The figure shows three views and two pictorial views of one solid part (mm, origin at its lowest corner). Answer the questions. A direction names the side the tool comes from. Round coordinates to 2 decimals unless told otherwise and drop trailing zeros. Order: outer loops, then holes, each group sorted by start corner. A loop starts at its lowest first (then second) coordinate and runs counter-clockwise, first axis right, second up. Notation, with made-up numbers: (38, 79) - (46, 79) arc R13 cw to (46, 95) - close; hole circle Ø5 at (77.5, 38). An arc over 180 degrees is marked (long way). Write item = value, one per line.
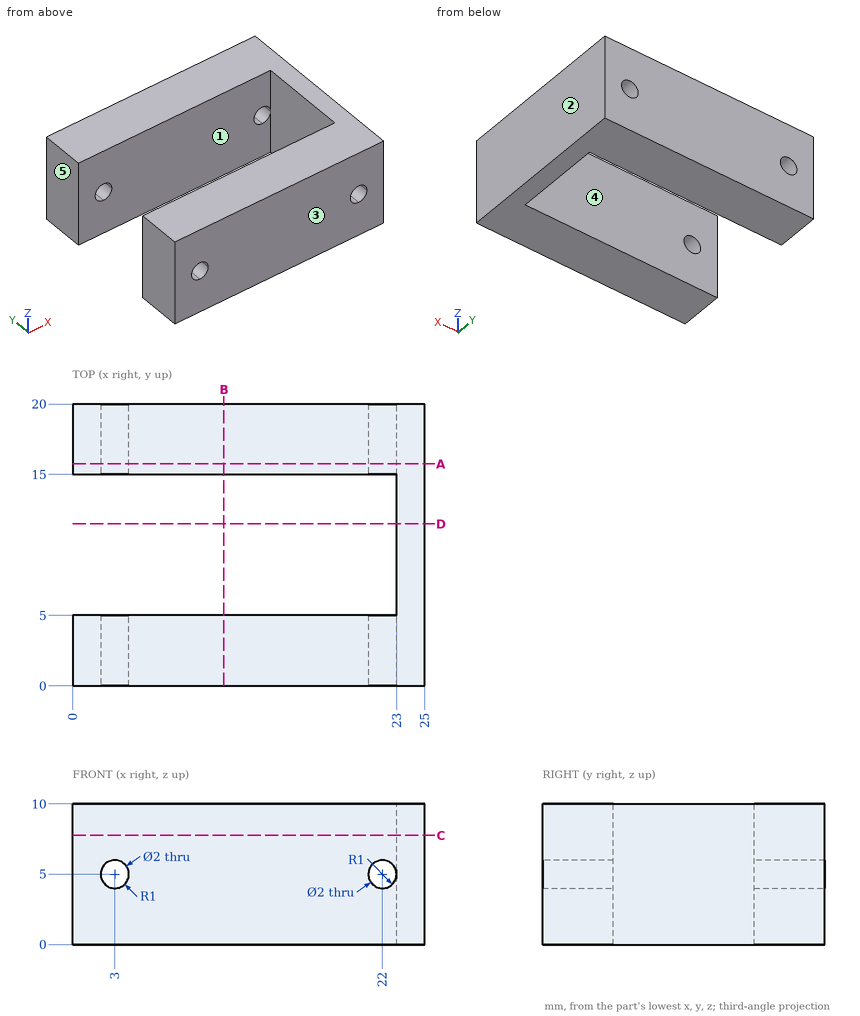
Q1. Determine the mould class of the marked faces 3, 4 and 5 for opening direction Y: released by +Y, released by -Y, zero draft, split by the parting line, or undercut.
Model answer:
face_3 = released by -Y
face_4 = undercut
face_5 = zero draft
Q2. Section A-A on y = 15.75 is taken. Determine the outline of the cut face in (x, z).
Model answer:
outline = (0, 0) - (25, 0) - (25, 10) - (0, 10) - close; hole circle Ø2 at (3, 5); hole circle Ø2 at (22, 5)
Q3. Find the intervals of material crossed by line 1 (X direction, y = 2.4, z = 5); line 2 (Y direction, x = 2.75, z = 7.5); line 3 (Z direction, x = 3, y = 1.5), in increasing order. Write a range as from..to.
Model answer:
line_1 = 0..2, 4..21, 23..25
line_2 = 0..5, 15..20
line_3 = 0..4, 6..10
Q4. A flat-ended cylindrical pin translates along its axis: P1, Ø1.8, axis at x = 22, z = 5, coming from the -Y side (3 decimals). Find the tip coordinate at first contact, or state that the pin passes through.
Model answer:
P1 = through
Q5. Section D-D on y = 11.5 is taken. Determine the outline of the cut face in (x, z).
Model answer:
outline = (23, 0) - (25, 0) - (25, 10) - (23, 10) - close
Q6. Section C-C on z = 7.75 is taken. Determine the outline of the cut face in (x, y), then the cut area to 3 significant figures.
Model answer:
outline = (0, 0) - (25, 0) - (25, 20) - (0, 20) - (0, 15) - (23, 15) - (23, 5) - (0, 5) - close
area = 270 mm^2
Q7. For the marked faces 1 and 2, determine the directions among +Z, -Z, +X, -X, +Y, -Y from which every point of the face is accessible in a straight line to the end or side of a thin tool.
Model answer:
face_1 = +Z, -Z, -X
face_2 = +Z, -Z, +X, +Y, -Y
Q8. Section B-B on x = 10.75 is taken. Determine the outline of the cut face in (y, z).
Model answer:
outline = (0, 0) - (5, 0) - (5, 10) - (0, 10) - close; (15, 0) - (20, 0) - (20, 10) - (15, 10) - close
